Can you work these out from the model? Positions are in its coordinate system, mm. A direction names the side the tool comes from. Round coordinates to 2 decimals unless told otherwise and drop trailing zeros. Loops run counter-clockwise (first coordinate to the right, second up) from the corner with the lowest first, then second, coordinate; pieces in that order, holes last. Notation, with made-up numbers: (-24, -13.5) -> (5, -13.5) arc R19 ccw to (5, 10.5) -> close; hole circle Ø8 at (-39.5, 53). An arc over 180 degrees is marked (long way). Use a Markdown table: item, result.
from build123d import *

# Parameters (mm, degrees)
F0_W      = 30
F0_H      = 30
F1_DEPTH  = 10
F2_W      = 10
F2_H      = 30
F3_DEPTH  = 20
F5_D      = 2
F5_DEPTH  = 20
F5_TIP    = 0.600860619
F7_D      = 3
F7_DEPTH  = 20
F7_TIP    = 0.9012909285
F9_D      = 4
F9_DEPTH  = 20
F9_TIP    = 1.2017212381
F11_D     = 5
F11_DEPTH = 20
F11_TIP   = 1.5021515476
F13_D     = 1.5
F13_DEPTH = 20
F13_TIP   = 0.4506454643
F15_D     = 2.5
F15_DEPTH = 20
F15_TIP   = 0.7510757738
F17_D     = 3.5
F17_DEPTH = 20
F17_TIP   = 1.0515060833
F19_D     = 4.5
F19_DEPTH = 20
F19_TIP   = 1.3519363928
F21_D     = 5.5
F21_DEPTH = 20
F21_TIP   = 1.6523667023
F22_DEPTH = 20
F23_SIZE  = 9.99999
F24_R     = 1
F25_DEPTH = 25
F26_R     = 1.5
F27_DEPTH = 25
F28_R     = 0.5
F29_DEPTH = 25
F31_DEPTH = 25
F33_DEPTH = 25
F34_W     = 5
F34_H     = 5
F35_DEPTH = 10
F36_W     = 5
F36_H     = 5
F37_DEPTH = 25


# Not quite as in the source:
# - a fillet or chamfer is up to 0.001 mm smaller than in the source, because OpenCascade refuses the exact size


with BuildPart() as f1:
    # F0 (on Top) → F1 (new body)
    with BuildSketch(Plane.XY):
        with Locations((15, 15)):
            Rectangle(F0_W, F0_H)
    extrude(amount=F1_DEPTH)

    # F2 (on face) → F3 (join)
    with BuildSketch(Plane.XY.offset(10)):
        with Locations((5, 15)):
            Rectangle(F2_W, F2_H)
    extrude(amount=F3_DEPTH)

    # F5
    with Locations(Plane.XY.offset(10)):
        with Locations((25, 5)):
            Hole(F5_D / 2, depth=F5_DEPTH)
            with Locations((0, 0, -(F5_DEPTH + F5_TIP / 2))):  # 118° drill point
                Cone(0, F5_D / 2, F5_TIP, mode=Mode.SUBTRACT)

    # F7
    with Locations(Plane.XY.offset(10)):
        with Locations((25, 10)):
            Hole(F7_D / 2, depth=F7_DEPTH)
            with Locations((0, 0, -(F7_DEPTH + F7_TIP / 2))):  # 118° drill point
                Cone(0, F7_D / 2, F7_TIP, mode=Mode.SUBTRACT)

    # F9
    with Locations(Plane.XY.offset(10)):
        with Locations((25, 15)):
            Hole(F9_D / 2, depth=F9_DEPTH)
            with Locations((0, 0, -(F9_DEPTH + F9_TIP / 2))):  # 118° drill point
                Cone(0, F9_D / 2, F9_TIP, mode=Mode.SUBTRACT)

    # F11
    with Locations(Plane.XY.offset(10)):
        with Locations((25, 22.5)):
            Hole(F11_D / 2, depth=F11_DEPTH)
            with Locations((0, 0, -(F11_DEPTH + F11_TIP / 2))):  # 118° drill point
                Cone(0, F11_D / 2, F11_TIP, mode=Mode.SUBTRACT)

    # F13
    with Locations(Plane.XY.offset(10)):
        with Locations((17.5, 5)):
            Hole(F13_D / 2, depth=F13_DEPTH)
            with Locations((0, 0, -(F13_DEPTH + F13_TIP / 2))):  # 118° drill point
                Cone(0, F13_D / 2, F13_TIP, mode=Mode.SUBTRACT)

    # F15
    with Locations(Plane.XY.offset(10)):
        with Locations((17.5, 10)):
            Hole(F15_D / 2, depth=F15_DEPTH)
            with Locations((0, 0, -(F15_DEPTH + F15_TIP / 2))):  # 118° drill point
                Cone(0, F15_D / 2, F15_TIP, mode=Mode.SUBTRACT)

    # F17
    with Locations(Plane.XY.offset(10)):
        with Locations((17.5, 15)):
            Hole(F17_D / 2, depth=F17_DEPTH)
            with Locations((0, 0, -(F17_DEPTH + F17_TIP / 2))):  # 118° drill point
                Cone(0, F17_D / 2, F17_TIP, mode=Mode.SUBTRACT)

    # F19
    with Locations(Plane.XY.offset(10)):
        with Locations((17.5, 20)):
            Hole(F19_D / 2, depth=F19_DEPTH)
            with Locations((0, 0, -(F19_DEPTH + F19_TIP / 2))):  # 118° drill point
                Cone(0, F19_D / 2, F19_TIP, mode=Mode.SUBTRACT)

    # F21
    with Locations(Plane.XY.offset(10)):
        with Locations((17.5, 26)):
            Hole(F21_D / 2, depth=F21_DEPTH)
            with Locations((0, 0, -(F21_DEPTH + F21_TIP / 2))):  # 118° drill point
                Cone(0, F21_D / 2, F21_TIP, mode=Mode.SUBTRACT)

    # F22 (cut): a face of the model
    f22_faces = [f1.faces().sort_by_distance(p)[0] for p in [
        (5, 15, 30),
    ]]
    extrude(f22_faces, amount=-F22_DEPTH, mode=Mode.SUBTRACT)

    # F23 (size 10 in the source; OpenCascade refuses exactly that, so slightly less here)
    f23_edges = [f1.edges().sort_by_distance(p)[0] for p in [
        (0, 15, 0),
    ]]
    chamfer(f23_edges, length=F23_SIZE)

    # F24 (on face) → F25 (join)
    with BuildSketch(Plane.XY.offset(10)):
        with Locations((10, 6)):
            Circle(F24_R)
    extrude(amount=F25_DEPTH)

    # F26 (on face) → F27 (join)
    with BuildSketch(Plane.XY.offset(10)):
        with Locations((10, 10)):
            Circle(F26_R)
    extrude(amount=F27_DEPTH)

    # F28 (on face) → F29 (join)
    with BuildSketch(Plane.XY.offset(10)):
        with Locations((10, 2.25)):
            Circle(F28_R)
    extrude(amount=F29_DEPTH)

    # F30 (on face) → F31 (join)
    with BuildSketch(Plane.XY.offset(10)):
        Polygon((12.1558459991, 16.8280467147), (10.3608135091, 18.2810407592), (8.20496751, 17.4529940445), (7.8441540009, 15.1719532853), (9.6391864909, 13.7189592408), (11.79503249, 14.5470059555), align=None)
    extrude(amount=F31_DEPTH)

    # F32 (on face) → F33 (join)
    with BuildSketch(Plane.XY.offset(10)):
        Polygon((13.8455249644, 22.8991195577), (9.0306279474, 27.8807625312), (7.1238470882, 21.2201179111), align=None)
    extrude(amount=F33_DEPTH)

    # F34 (on face) → F35 (join)
    with BuildSketch(Plane.YZ.offset(30)):
        with Locations((2.5, 7.5)):
            Rectangle(F34_W, F34_H)
        with Locations((27.5, 7.5)):
            Rectangle(F34_W, F34_H)
    extrude(amount=F35_DEPTH)

    # F36 (on face) → F37 (join)
    with BuildSketch(Plane.XZ.offset(-25)):
        with Locations((37.5, 7.5)):
            Rectangle(F36_W, F36_H)
    extrude(amount=F37_DEPTH)


solid = f1.part
1. I want a section at D-D (z = 4.5). State how many separate pieces and enclosed holes the cut face has, plus the area to 3 significant figures.
Answer sheet:
| item | result |
|---|---|
| separate pieces | 1 |
| enclosed holes | 9 |
| area | 637 mm² |
2. If we mould it in two halves opening along X, with no side actions, what happens to faces 1 (the cylindrical face through (26.5, 10.07, 4.93)), 2 (the flat face through (11.271, 17.544, 22.325)), 3 (the flat face through (20, 15, 0))? For each: +X half, -X half, draft (parallel to the pull), parting line (faces both ways), or undercut.
Answer sheet:
| item | result |
|---|---|
| face 1 | undercut |
| face 2 | +X half |
| face 3 | draft |
3. Will these pins go through, and if not, where does the flat tip stop? pin 1 Ø4 at (y, z) = (16.5, 19.5) entering from -X; pin 2 Ø6 at (x, y) = (17.5, 20) entering from +Z; pin 3 Ø1.5 at (y, z) = (6, 29.5) entering from -X.
Answer sheet:
| item | result |
|---|---|
| pin 1 | stops at x = 7.84 |
| pin 2 | stops at z = 10 |
| pin 3 | stops at x = 9 |
4. I want a section at B-B (z = 21.5). Please give me the cut outline in (x, y).
Answer sheet:
| item | result |
|---|---|
| outline | (7.12, 21.22) -> (13.85, 22.9) -> (9.03, 27.88) -> close; (7.84, 15.17) -> (9.64, 13.72) -> (11.8, 14.55) -> (12.16, 16.83) -> (10.36, 18.28) -> (8.2, 17.45) -> close; circle Ø3 at (10, 10); circle Ø2 at (10, 6); circle Ø1 at (10, 2.25) |
5. I want a section at A-A (x = 17.5). Please give me the cut outline in (y, z), plus the area to 3 significant figures.
Answer sheet:
| item | result |
|---|---|
| outline | (0, 0) -> (4.25, 0) -> (4.25, 10) -> (0, 10) -> close; (5.75, 0) -> (8.75, 0) -> (8.75, 10) -> (5.75, 10) -> close; (11.25, 0) -> (13.25, 0) -> (13.25, 10) -> (11.25, 10) -> close; (16.75, 0) -> (17.75, 0) -> (17.75, 10) -> (16.75, 10) -> close; (22.25, 0) -> (23.25, 0) -> (23.25, 10) -> (22.25, 10) -> close; (28.75, 0) -> (30, 0) -> (30, 10) -> (28.75, 10) -> close |
| area | 125 mm² |
6. I want a section at C-C (x = 25). Please give me the cut outline in (y, z), plus the area to 3 significant figures.
Answer sheet:
| item | result |
|---|---|
| outline | (0, 0) -> (4, 0) -> (4, 10) -> (0, 10) -> close; (6, 0) -> (8.5, 0) -> (8.5, 10) -> (6, 10) -> close; (11.5, 0) -> (13, 0) -> (13, 10) -> (11.5, 10) -> close; (17, 0) -> (20, 0) -> (20, 10) -> (17, 10) -> close; (25, 0) -> (30, 0) -> (30, 10) -> (25, 10) -> close |
| area | 160 mm² |
7. I need wall thicknesses on line 1 (Y direction, x = 17.5, z = 6.25); line 2 (Y direction, x = 25, z = 5); line 3 (Y direction, x = 17, z = 7). Which ranges of each line are inside material? Lowest first, please.
Answer sheet:
| item | result |
|---|---|
| line 1 | y = 0 to 4.25, 5.75 to 8.75, 11.25 to 13.25, 16.75 to 17.75, 22.25 to 23.25, 28.75 to 30 |
| line 2 | y = 0 to 4, 6 to 8.5, 11.5 to 13, 17 to 20, 25 to 30 |
| line 3 | y = 0 to 4.44, 5.56 to 8.85, 11.15 to 13.32, 16.68 to 17.81, 22.19 to 23.3, 28.7 to 30 |
8. Which directions (+Z, -Z, +X, -X, +Y, -Y) give clear straight access to the entire face, cutting with the end or side of a thin tool? Please do faces 4 (the flat face through (11.472, 25.355, 22.325)), 5 (the flat face through (32, 5, 7)), 6 (the flat face through (30, 15, 5)), 7 (the flat face through (11.973, 15.672, 22.325)), 8 (the cylindrical face through (8.8, 9.1, 22.3)).
Answer sheet:
| item | result |
|---|---|
| face 4 | +Z, +X, +Y |
| face 5 | +Z, -Z |
| face 6 | -Z |
| face 7 | +Z, +X, -Y |
| face 8 | +Z |
